Can you work these out from the drawing? Everything is in mm from the part's minimum corner. A direction names the side the tool comes from. Coordinates: 2 decimals unless noted, no trailing zeros. Loops run counter-clockwise (first coordinate to the right, second up) from the corner with the lowest first, then second, coordinate; pieces in that order, holes last.
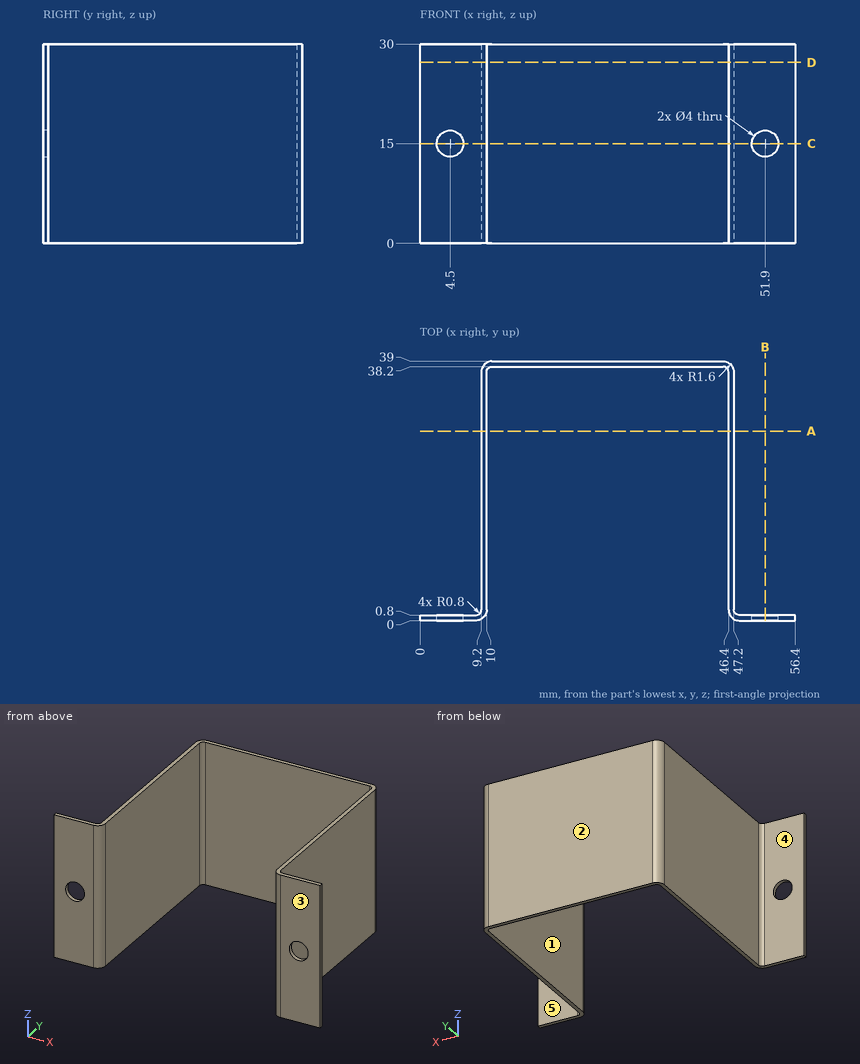
Item 1: Suppose I cut it at C-C, the plane z = 15. Please give me the cut outline in (x, y), plus the area to 3 significant figures.
Results are:
outline: (0, 0) - (2.5, 0) - (2.5, 0.8) - (0, 0.8) - close; (6.5, 0) - (8.4, 0) arc R1.6 ccw to (10, 1.6) - (10, 37.4) arc R0.8 cw to (10.8, 38.2) - (45.6, 38.2) arc R0.8 cw to (46.4, 37.4) - (46.4, 1.6) arc R1.6 ccw to (48, 0) - (49.9, 0) - (49.9, 0.8) - (48, 0.8) arc R0.8 cw to (47.2, 1.6) - (47.2, 37.4) arc R1.6 ccw to (45.6, 39) - (10.8, 39) arc R1.6 ccw to (9.2, 37.4) - (9.2, 1.6) arc R0.8 cw to (8.4, 0.8) - (6.5, 0.8) - close; (53.9, 0) - (56.4, 0) - (56.4, 0.8) - (53.9, 0.8) - close
area: 98.2 mm2
Item 2: Suppose I cut it at D-D, the plane z = 27.25. Please give me the cut outline in (x, y).
Results are:
outline: (0, 0) - (8.4, 0) arc R1.6 ccw to (10, 1.6) - (10, 37.4) arc R0.8 cw to (10.8, 38.2) - (45.6, 38.2) arc R0.8 cw to (46.4, 37.4) - (46.4, 1.6) arc R1.6 ccw to (48, 0) - (56.4, 0) - (56.4, 0.8) - (48, 0.8) arc R0.8 cw to (47.2, 1.6) - (47.2, 37.4) arc R1.6 ccw to (45.6, 39) - (10.8, 39) arc R1.6 ccw to (9.2, 37.4) - (9.2, 1.6) arc R0.8 cw to (8.4, 0.8) - (0, 0.8) - close
Item 3: Suppose I cut it at B-B, the plane x = 51.9. Please give me the cut outline in (y, z).
Results are:
outline: (0, 0) - (0.8, 0) - (0.8, 13) - (0, 13) - close; (0, 17) - (0.8, 17) - (0.8, 30) - (0, 30) - close
Item 4: Suppose I cut it at A-A, the plane y = 28.5. Please give me the cut outline in (x, z), plus the area to 3 significant figures.
Results are:
outline: (9.2, 0) - (10, 0) - (10, 30) - (9.2, 30) - close; (46.4, 0) - (47.2, 0) - (47.2, 30) - (46.4, 30) - close
area: 48.0 mm2
Item 5: On a 3-axis mill with a long thin cutter (end or side, diameter ignored), from which of +Z, -Z, +X, -X, +Y, -Y can I reach the whole of each face in a straight line? I mean the marked faces 1, 2, 3, 4 and 5. Say none if no direction works.
Results are:
face 1: +Z, -Z, -Y
face 2: +Z, -Z, +X, -X, +Y
face 3: +Z, -Z, +X, -X, -Y
face 4: +Z, -Z, -X, +Y
face 5: +Z, -Z, +X, +Y
Item 6: I need wall thicknesses on line 1 along X through (y, z) = (37.5, 3); line 2 along X through (y, z) = (0.2, 15); line 3 along X through (y, z) = (0.3, 15). Which ranges of each line are inside material? Lowest first, please.
Results are:
line 1: x = 9.2 to 10.01, 46.39 to 47.2
line 2: x = 0 to 2.5, 6.5 to 9.17, 47.23 to 49.9, 53.9 to 56.4
line 3: x = 0 to 2.5, 6.5 to 9.33, 47.07 to 49.9, 53.9 to 56.4
Item 7: I'm going to push flat-ended pins straight in: P1, Ø15, axis at y = 12.5, z = 20.5, coming from the +X side; P2, Ø3, axis at x = 4.5, z = 15, coming from the +Y side; P3, Ø5, axis at x = 11, z = 14.5, coming from the -Y side; P4, Ø10, axis at x = 25, z = 14, coming from the -Y side. Where does each tip first touch, or does it pass through?
Results are:
P1: stops at x = 47.2
P2: passes through
P3: stops at y = 0
P4: stops at y = 38.2
